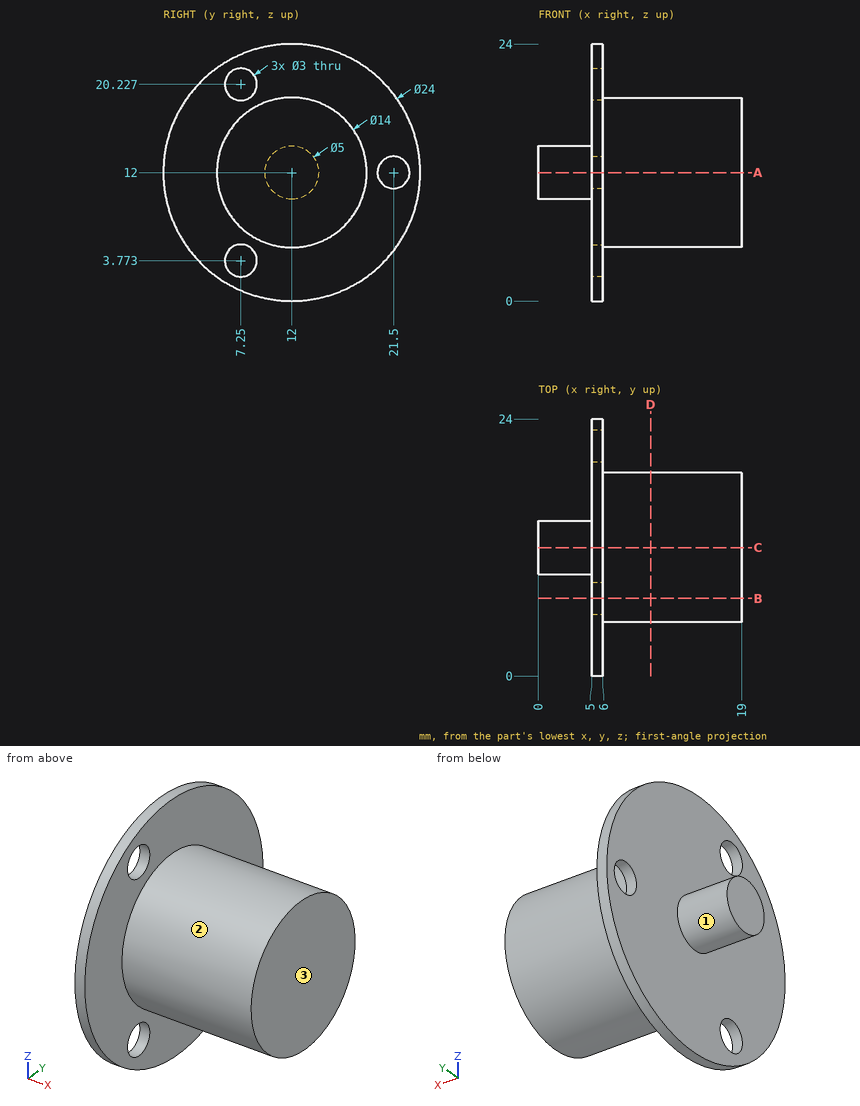
Study the drawing (mm; zero at the part's minimum x, y, z) and answer. A direction names the side the tool comes from. Round coordinates to 2 decimals unless told otherwise and drop trailing zeros. Write each loop counter-clockwise with the first axis right and the second up, starting at its lowest first coordinate (ties: lowest second). Pieces come first, ordered by that corner, then holes. Notation, with made-up numbers: (23.5, 22) -> (41.5, 22) arc R24 cw to (41.5, 32) -> close; hole circle Ø8 at (50, 79.25). An arc over 180 degrees is marked (long way). Answer as CSV lines item,"result". Start each with the question number.
(1) The part is cut by section D-D, the plane x = 10.5. Give the vertices of the cut face in (y, z), then the cut area to 3 significant figures.
(2) Find the intervals of material crossed by probe 1 along Y at (x, z) = (17.5, 11.75); probe 2 along Y at (x, z) = (5.5, 12); probe 3 along Y at (x, z) = (3.75, 12), in increasing order.
(3) The part is cut by section C-C, the plane y = 12. Give the vertices of the cut face in (x, z), then the cut area to 3 significant figures.
(4) The part is cut by section B-B, the plane y = 7.25. Give the vertices of the cut face in (x, z), then the cut area to 3 significant figures.
(5) Each of these flat-tipped pins is pushed along its axis until it touches: pin 1 (4 mm diameter, centred on y = 19, z = 17, fed in from -X); pin 2 (8 mm diameter, centred on x = 16, z = 21, fed in from -Y); pin 3 (2.5 mm diameter, centred on y = 7.25, z = 3.77, fed in from -X); pin 4 (5 mm diameter, centred on x = 14.5, y = 17, fed in from -Z). Where does it stop, or does it pass through?
(6) The part is cut by section A-A, the plane z = 12. Give the vertices of the cut face in (x, y).
(7) A tool of negligible diameter and unlimited length cuts with its end or side. For the marked faces 1, 2 and 3, from which of +Z, -Z, +X, -X, +Y, -Y can it reach the whole face along a straight path? Write none if from no direction.
Output values:
1,outline,"circle Ø14 at (12, 12)"
1,area,"154 mm²"
2,probe 1,"y = 5 to 19"
2,probe 2,"y = 0 to 20, 23 to 24"
2,probe 3,"y = 9.5 to 14.5"
3,outline,"(0, 9.5) -> (5, 9.5) -> (5, 0) -> (6, 0) -> (6, 5) -> (19, 5) -> (19, 19) -> (6, 19) -> (6, 24) -> (5, 24) -> (5, 14.5) -> (0, 14.5) -> close"
3,area,"231 mm²"
4,outline,"(5, 0.98) -> (6, 0.98) -> (6, 2.27) -> (5, 2.27) -> close; (5, 5.27) -> (6, 5.27) -> (6, 6.86) -> (19, 6.86) -> (19, 17.14) -> (6, 17.14) -> (6, 18.73) -> (5, 18.73) -> close; (5, 21.73) -> (6, 21.73) -> (6, 23.02) -> (5, 23.02) -> close"
4,area,"150 mm²"
5,pin 1,"stops at x = 5"
5,pin 2,"stops at y = 7.1"
5,pin 3,"passes through"
5,pin 4,"stops at z = 5.46"
6,outline,"(0, 9.5) -> (5, 9.5) -> (5, 0) -> (6, 0) -> (6, 5) -> (19, 5) -> (19, 19) -> (6, 19) -> (6, 20) -> (5, 20) -> (5, 14.5) -> (0, 14.5) -> close; (5, 23) -> (6, 23) -> (6, 24) -> (5, 24) -> close"
7,face 1,"-X"
7,face 2,"+X"
7,face 3,"+Z, -Z, +X, +Y, -Y"
